For this review, take the finished solid that the model builds, in its own axes (mm). Face numbers are marked on the shaded views. A direction names the side the tool comes from. Coordinates: 2 decimals unless noted, no trailing zeros. Write each loop counter-clockwise with the first axis right and the second up, starting at its lowest first coordinate (ties: lowest second). Pieces come first, ordered by that corner, then holes. Notation, with made-up numbers: M -23,19 L 24,19 A13 ccw 24,42 Z; hole C 56,18.5 d4. An arc over 180 degrees is marked long. Return JSON: item names as keys, results as strings.
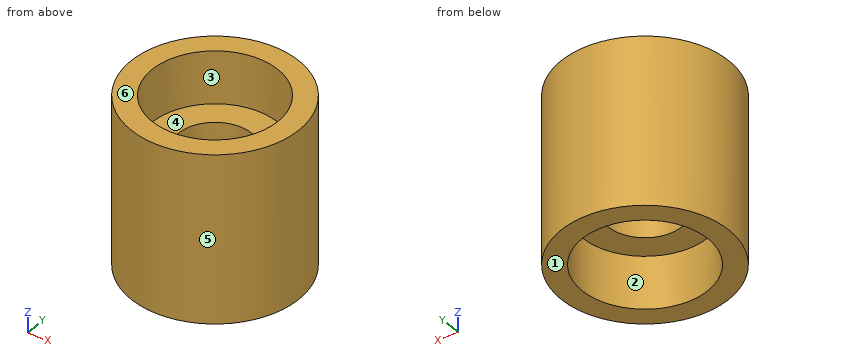
Autodesk Fusion 360 part; units mm, degrees
sketch "Sketch1" plane through (0, 0, 0) normal (0, 0, 1) x (1, 0, 0)
  circle A0 centre (0, 0) radius 1.75
  circle A1 centre (0, 0) radius 3
  circle A2 centre (0, 0) radius 4
  dimension "d1" = 3.5
  dimension "d2" = 6
  dimension "d3" = 8
extrude "Extrude1" add sketch "Sketch1" against normal blind 3 contours A1
extrude "Extrude2" add sketch "Sketch1" along normal blind 2.5 and the other way blind 5.5 contours A2
1. We need section D-D (x = -2.25). State the section outline as (y, z) points.
Checks:
{"outline": "M -3.31,-5.5 L -1.98,-5.5 L -1.98,-3 L 1.98,-3 L 1.98,-5.5 L 3.31,-5.5 L 3.31,2.5 L 1.98,2.5 L 1.98,0 L -1.98,0 L -1.98,2.5 L -3.31,2.5 Z"}
2. For the marked faces 1, 2 and 3, list the 3-axis set-ups (+Z, -Z, +X, -X, +Y, -Y) from which the entire face can be reached by the end or side of a thin tool; tool diameter is ignored.
Checks:
{"face 1": "-Z, +X, -X, +Y, -Y", "face 2": "-Z", "face 3": "+Z"}
3. Draft analysis for pull direction Y (two halves, no side actions). For the marked faces 4, 5 and 6, state which applies: +Y half, -Y half, draft (parallel to the pull), parting line (faces both ways), or undercut.
Checks:
{"face 4": "undercut", "face 5": "parting line", "face 6": "draft"}
4. Wall thickness on L1, parallel to Y at x = 0, z = 2; L2, parallel to Y at x = 0, z = -1.8; L3, parallel to X at y = 0.5, z = -0.25: over which ranges is each line inside the solid? List them lowest first. Write a range as from..to.
Checks:
{"L1": "-4..-3, 3..4", "L2": "-4..-1.75, 1.75..4", "L3": "-3.97..-1.68, 1.68..3.97"}
5. Clearance check with flat-ended pins moving along their axes: pin 1 Ø4 at (x, y) = (0, 0) entering from +Z; pin 2 Ø1.5 at (y, z) = (2.5, -4.5) entering from +X. State where each tip first meets the part, or that it passes through.
Checks:
{"pin 1": "z = 0", "pin 2": "x = 3.6"}
6. We need section C-C (z = -4.5). State the section outline as (x, y) points, plus the area to 3 significant figures.
Checks:
{"outline": "C 0,0 d8; hole C 0,0 d6", "area": "22.0 mm2"}
7. We need section A-A (y = 0). State the section outline as (x, z) points, plus the area to 3 significant figures.
Checks:
{"outline": "M -4,-5.5 L -3,-5.5 L -3,-3 L -1.75,-3 L -1.75,0 L -3,0 L -3,2.5 L -4,2.5 Z; M 1.75,-3 L 3,-3 L 3,-5.5 L 4,-5.5 L 4,2.5 L 3,2.5 L 3,0 L 1.75,0 Z", "area": "23.5 mm2"}
